```python
from build123d import *

# Parameters (mm, degrees)
SKETCH1_W             = 103.1748
SKETCH1_H             = 32.766
TRS_PCB_DEPTH         = 1.4605
SKETCH2_R             = 1.4859
STAND_OFF_HOLES_DEPTH = 1.4605
SKETCH3_W             = 14.732
SKETCH3_H             = 14.732
GPS_ANTENNA_DEPTH     = 6.604
SKETCH4_W             = 6.35
SKETCH4_H             = 6.096
BOSS_EXTRUDE2_DEPTH   = 1.27
SKETCH5_R             = 5.334
BOSS_EXTRUDE3_DEPTH   = 15.24
BOSS_EXTRUDE3_TAPER   = 5
SKETCH6_R             = 4.0005
BOSS_EXTRUDE4_DEPTH   = 96.774


with BuildPart() as part:
    # Sketch1 → TRS PCB (new body)
    with BuildSketch(Plane(origin=(0, 0, 0), x_dir=(1, 0, 0), z_dir=(0, 1, 0))):
        Rectangle(SKETCH1_W, SKETCH1_H)
    extrude(amount=TRS_PCB_DEPTH)

    # Sketch2 → Stand off holes (cut)
    with BuildSketch(Plane(origin=(0, 1.4605, 0), x_dir=(1, 0, 0), z_dir=(0, 1, 0))):
        with Locations((-49.3395, 14.1351)):
            Circle(SKETCH2_R)
        with Locations((49.3395, 14.1351)):
            Circle(SKETCH2_R)
        with Locations((49.3395, -14.1351)):
            Circle(SKETCH2_R)
        with Locations((-49.3395, -14.1351)):
            Circle(SKETCH2_R)
    extrude(amount=-STAND_OFF_HOLES_DEPTH, mode=Mode.SUBTRACT)

    # Sketch3 → GPS Antenna (add)
    with BuildSketch(Plane(origin=(0, 1.4605, 0), x_dir=(1, 0, 0), z_dir=(0, 1, 0))):
        with Locations((13.7414, 5.207)):
            Rectangle(SKETCH3_W, SKETCH3_H)
    extrude(amount=GPS_ANTENNA_DEPTH)

    # Sketch4 → Boss-Extrude2 (add)
    with BuildSketch(Plane.ZY.offset(51.5874)):
        with Locations((-1.27, 2.286)):
            Rectangle(SKETCH4_W, SKETCH4_H)
    extrude(amount=BOSS_EXTRUDE2_DEPTH)

    # Sketch5 → Boss-Extrude3 (add)
    with BuildSketch(Plane.ZY.offset(52.8574)):
        with Locations((-1.27, 2.286)):
            Circle(SKETCH5_R)
    extrude(amount=BOSS_EXTRUDE3_DEPTH, taper=BOSS_EXTRUDE3_TAPER)

    # Sketch6 → Boss-Extrude4 (add)
    with BuildSketch(Plane.ZY.offset(68.0974)):
        with Locations((-1.27, 2.286)):
            Circle(SKETCH6_R)
    extrude(amount=BOSS_EXTRUDE4_DEPTH)


solid = part.part
```
Geometry: final body of the model. Coordinates: model frame, mm. A direction names the side the tool comes from. Coordinates: 2 decimals unless noted, no trailing zeros. Loops run counter-clockwise (first coordinate to the right, second up) from the corner with the lowest first, then second, coordinate; pieces in that order, holes last. Notation, with made-up numbers: (60.25, -31.75) -> (93.25, -31.75) arc R18 ccw to (93.25, -10.75) -> close; hole circle Ø4 at (8.5, 19.5). An arc over 180 degrees is marked (long way). Use a Markdown table: item, result. Add a question column.
(1) Section query B-B, the plane x = -15.5. Return loops of the section in (y, z), plus the area to 3 significant figures.
(2) Section query C-C, the plane z = -9. Return loops of the section in (x, y).
(3) Line query: line 1 along X through (y, z) = (2, 0.5); line 2 along Z through (x, y) = (8.5, 5.75); line 3 along X through (y, z) = (-0.5, -1). Output: solid intervals per line, ascending.
(4) Mould query, pull axis X, two halves, no side actions, for faces 5 (the flat face through (14, 5, 2.159)), 6 (the flat face through (-52.857, 2.4, 2.2)), 7 (the flat face through (-164.871, 2, -1)). Classes: pulls with the +X half, pulls with the -X half, needs draft (parallel to the pull), parting line crosses it, or undercut.
(5) Access query for faces 1 (the cylindrical face through (-115.807, -0.148, -4.445)), 2 (the flat face through (14, 5, -12.573)), 3 (the flat face through (-1, 0, 0)), 4 (the flat face through (-51.587, 3, -1)). Directions: +Z, -Z, +X, -X, +Y, -Y. A direction counts if a zero-diameter tool reaches every point of the face in a straight line with its end or side. Return the directions, or none.
(6) Pin query (flat end, axial travel): pin 1 Ø10 at (x, z) = (14, 4) entering from -Y; pin 2 Ø0.6 at (x, y) = (-52, 3) entering from +Z (3 decimals); pin 3 Ø4 at (x, y) = (-132.5, 2.5) entering from -Z; pin 4 Ø1.8 at (x, z) = (49.34, -14.14) entering from +Y. Return the tip coordinate at first contact, or that it passes through.
(7) Section query D-D, the plane z = 8. Return loops of the section in (x, y), plus the area to 3 significant figures.
Answer:
| question | item | result |
|---|---|---|
| 1 | outline | (0, -16.38) -> (1.46, -16.38) -> (1.46, 16.38) -> (0, 16.38) -> close |
| 1 | area | 47.9 mm^2 |
| 2 | outline | (-51.59, 0) -> (51.59, 0) -> (51.59, 1.46) -> (21.11, 1.46) -> (21.11, 8.06) -> (6.38, 8.06) -> (6.38, 1.46) -> (-51.59, 1.46) -> close |
| 3 | line 1 | x = -164.87 to -51.59, 6.38 to 21.11 |
| 3 | line 2 | z = -12.57 to 2.16 |
| 3 | line 3 | x = -164.87 to -51.59 |
| 4 | face 5 | needs draft |
| 4 | face 6 | undercut |
| 4 | face 7 | pulls with the -X half |
| 5 | face 1 | -X |
| 5 | face 2 | -Z, +X, -X, +Y |
| 5 | face 3 | +Z, -Z, +X, -Y |
| 5 | face 4 | +Z, -Z, +Y |
| 6 | pin 1 | stops at y = 0 |
| 6 | pin 2 | stops at z = 1.905 |
| 6 | pin 3 | stops at z = -5.27 |
| 6 | pin 4 | passes through |
| 7 | outline | (-51.59, 0) -> (51.59, 0) -> (51.59, 1.46) -> (-51.59, 1.46) -> close |
| 7 | area | 151 mm^2 |
